from build123d import *

# Parameters (mm, degrees)
SKETCH019_W     = 10
SKETCH019_H     = 3
PAD011_DEPTH    = 3
POCKET007_DEPTH = 5
CHAMFER004_SIZE = 0.4


with BuildPart() as part:
    # Sketch019 → Pad011 (new body)
    with BuildSketch(Plane.XY):
        with Locations((5, 0)):
            Rectangle(SKETCH019_W, SKETCH019_H)
    extrude(amount=PAD011_DEPTH)

    # Sketch020 (on Face1 of Pad011) → Pocket007 (cut)
    with BuildSketch(Plane(origin=(0, 1.5, 0), x_dir=(-1, 0, 0), z_dir=(0, 1, 0))):
        Polygon((0, 0.8), (-6.4, 3), (0, 3), align=None)
    extrude(amount=-POCKET007_DEPTH, mode=Mode.SUBTRACT)

    # Chamfer004
    chamfer004_edges = [part.edges().sort_by_distance(p)[0] for p in [
        (3.2, 1.5, 1.9),
        (3.2, -1.5, 1.9),
    ]]
    chamfer(chamfer004_edges, length=CHAMFER004_SIZE)


solid = part.part
Work out the finished part from the listing and answer in its coordinate system (mm). Coordinates: 2 decimals unless noted, no trailing zeros. Write each loop counter-clockwise with the first axis right and the second up, starting at its lowest first coordinate (ties: lowest second). Pieces come first, ordered by that corner, then holes. Notation, with made-up numbers: (-36, 1) - (18, 1) arc R19 cw to (18, 16) - close; hole circle Ø10 at (-39.5, 65.5). An arc over 180 degrees is marked (long way). One line per question, with ' | ' between items.
1) Find section C-C, the plane x = 4.5. Determine the outline of the cut face in (y, z).
Checks:
outline: (-1.5, 0) - (1.5, 0) - (1.5, 1.92) - (1.1, 2.35) - (-1.1, 2.35) - (-1.5, 1.92) - close
2) Consider probe 1 along Z at (x, y) = (2, -1.2); probe 2 along Z at (x, y) = (1.5, 1.25). Determine where each line is inside the solid, lowest interval first. Write a range as [from, to].
Checks:
probe 1: [0, 1.38] | probe 2: [0, 1.16]
3) A flat-ended cylindrical pin translates along its axis: P1, Ø1.5, axis at x = 1.5, y = 1, coming from the -Z side. Find the tip coordinate at first contact, or state that the pin passes through.
Checks:
P1: z = 0
4) Find section B-B, the plane z = 1.1. Determine the outline of the cut face in (x, y).
Checks:
outline: (0.87, -1.1) - (2.1, -1.5) - (10, -1.5) - (10, 1.5) - (2.1, 1.5) - (0.87, 1.1) - close
5) Find section A-A, the plane y = -0.25. Determine the outline of the cut face in (x, z), and give its area (3 significant figures).
Checks:
outline: (0, 0) - (10, 0) - (10, 3) - (6.4, 3) - (0, 0.8) - close | area: 23.0 mm2
